from build123d import *

# Parameters (mm, degrees)
F0_R     = 19.05
F1_DEPTH = 12.7
F3_DEPTH = 6.35
F4_R     = 3.96875
F5_DEPTH = 6.351
F6_SIZE  = 5.08


with BuildPart() as f1:
    # F0 (on Top) → F1 (new body)
    with BuildSketch(Plane.XY):
        Circle(F0_R)
    extrude(amount=F1_DEPTH)

    # F2 (on face) → F3 (cut)
    with BuildSketch(Plane.XY.offset(12.7)):
        Polygon((6.6843, -0.908523), (4.128954, 5.334513), (-2.555347, 6.243035), (-6.6843, 0.908523), (-4.128954, -5.334513), (2.555347, -6.243035), align=None)
    extrude(amount=-F3_DEPTH, mode=Mode.SUBTRACT)

    # F4 (on face) → F5 (cut, through all)
    with BuildSketch(Plane.XY.offset(6.35)):
        Circle(F4_R)
    extrude(amount=-F5_DEPTH, mode=Mode.SUBTRACT)

    # F6
    f6_edges = [f1.edges().sort_by_distance(p)[0] for p in [
        (-19.05, 0, 12.7),
    ]]
    chamfer(f6_edges, length=F6_SIZE)


solid = f1.part
Part model, mm, in its own coordinate system. A direction names the side the tool comes from. Coordinates: 2 decimals unless noted, no trailing zeros. Write each loop counter-clockwise with the first axis right and the second up, starting at its lowest first coordinate (ties: lowest second). Pieces come first, ordered by that corner, then holes. Notation, with made-up numbers: M 21,-9.75 L 33,-9.75 A34 cw 33,25.25 Z; hole C 66.5,68.5 d6. An arc over 180 degrees is marked long. Return JSON: item names as keys, results as strings.
1. Saw through at C-C, the plane y = 0. Write the cut outline in (x, z).
Determined:
{"outline": "M -19.05,0 L -3.97,0 L -3.97,6.35 L -6.31,6.35 L -6.31,12.7 L -13.97,12.7 L -19.05,7.62 Z; M 3.97,0 L 19.05,0 L 19.05,7.62 L 13.97,12.7 L 6.31,12.7 L 6.31,6.35 L 3.97,6.35 Z"}
2. Saw through at A-A, the plane x = 0. Write the cut outline in (y, z), then the cut area to 3 significant figures.
Determined:
{"outline": "M -19.05,0 L -3.97,0 L -3.97,6.35 L -5.9,6.35 L -5.9,12.7 L -13.97,12.7 L -19.05,7.62 Z; M 3.97,0 L 19.05,0 L 19.05,7.62 L 13.97,12.7 L 5.9,12.7 L 5.9,6.35 L 3.97,6.35 Z", "area": "333 mm²"}
3. Flat gauge pins, fed straight in: pin 1 Ø2 at (x, z) = (7.5, 3) entering from -Y; pin 2 Ø6 at (x, y) = (-1.5, -1.5) entering from +Z; pin 3 Ø1.5 at (x, z) = (-3.5, 7.5) entering from -Y; pin 4 Ø7 at (x, y) = (0, 0) entering from +Z. Where does each tip first touch, or does it go through?
Determined:
{"pin 1": "y = -17.91", "pin 2": "z = 6.35", "pin 3": "y = -18.85", "pin 4": "through"}
4. Saw through at B-B, the plane z = 5.5. Write the cut outline in (x, y), then the cut area to 3 significant figures.
Determined:
{"outline": "C 0,0 d38.1; hole C 0,0 d7.94", "area": "1,090 mm²"}
5. Pull direction X, two halves, no side cores. Call faces 3 (the face through (3, -6, 12.7)), 4 (the face through (-15.12, -11.59, 3.76)), 5 (the face through (0.834, 5.782, 9.569)): pulls with the +X half, pulls with the -X half, needs draft (parallel to the pull), parting line crosses it, or undercut.
Determined:
{"face 3": "needs draft", "face 4": "parting line crosses it", "face 5": "undercut"}
6. 3-axis set-ups, long thin cutter, end or side, ignore diameter. For faces 1 (the face through (-5.425, -2.169, 9.569)), 2 (the face through (-0.86, -3.874, 3.219)): which of +Z, -Z, +X, -X, +Y, -Y reach the whole face in a straight line?
Determined:
{"face 1": "+Z", "face 2": "+Z, -Z"}
7. Probe L1, parallel to Y at x = 0, z = 5; L2, parallel to Y at x = 1, z = 7.5; L3, parallel to Z at x = -3, y = -3.5. List the from-to ranges inside material, lowest first.
Determined:
{"L1": "-19.05 to -3.97, 3.97 to 19.05", "L2": "-19.02 to -6.03, 5.76 to 19.02", "L3": "0 to 6.35"}
